Check sheet for the drawn part. Datum: minimum x, y, z corner. Units: mm. Coordinates: 2 decimals unless noted, no trailing zeros. Write each loop counter-clockwise with the first axis right and the second up, starting at its lowest first coordinate (ties: lowest second). Pieces come first, ordered by that corner, then holes. Notation, with made-up numbers: M 27.5,17 L 61.5,17 A19 cw 61.5,54 Z; hole C 84,51 d7. An arc over 180 degrees is marked long. Answer in a Markdown table with one row per item.
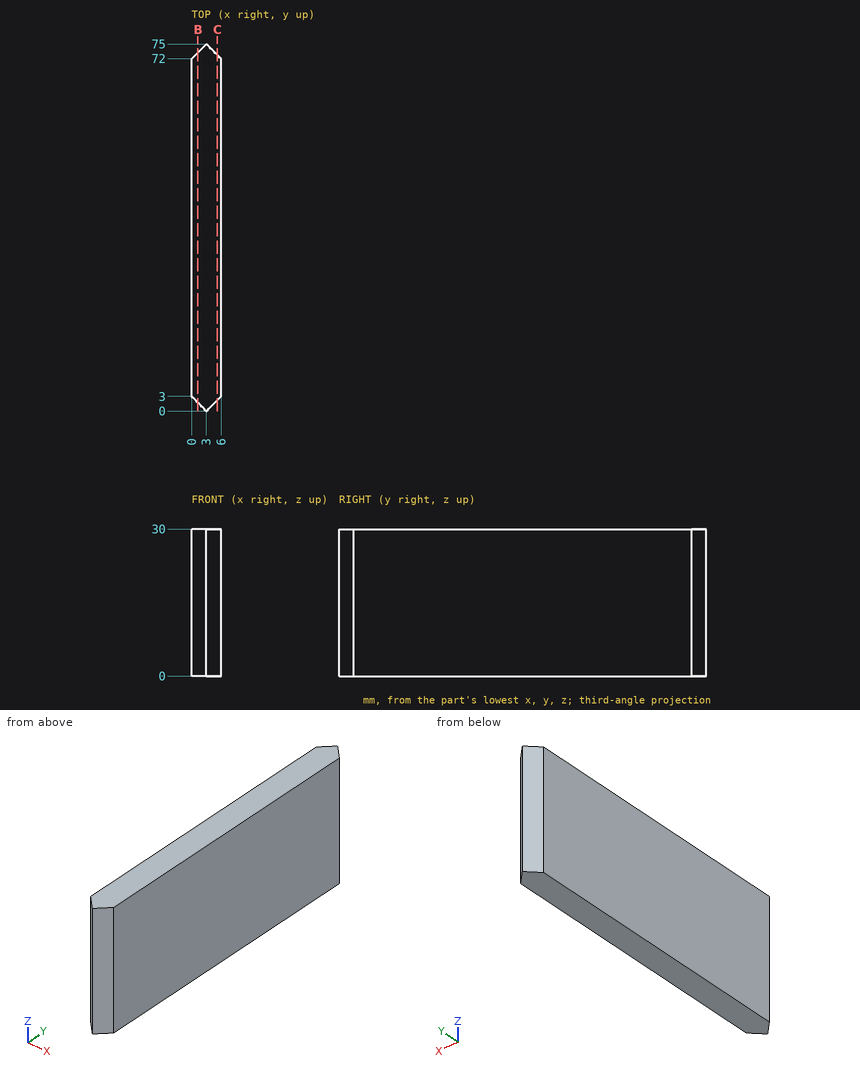
1) Sectioned sample at B-B (x = 1.25). Record the cut outline in (y, z).
Response values:
| item | result |
|---|---|
| outline | M 1.75,0 L 73.25,0 L 73.25,30 L 1.75,30 Z |
2) Depth check by flat-ended pin: pin 1 (3 mm diameter, centred on x = 3.5, z = 7.5, fed in from -Y). Enter the tip coordinate at first touch or a pass-through.
Response values:
| item | result |
|---|---|
| pin 1 | stops at y = 0 |
3) Sectioned sample at C-C (x = 5.25). Record the cut outline in (y, z), then the cut area to 4 significant figures.
Response values:
| item | result |
|---|---|
| outline | M 2.25,0 L 72.75,0 L 72.75,30 L 2.25,30 Z |
| area | 2,115 mm² |
4) Thickness scan on L1, parallel to Y at x = 1, z = 19; L2, parallel to Y at x = 2, z = 22. Record the ranges inside material, lowest first. Write a range as [from, to].
Response values:
| item | result |
|---|---|
| L1 | y = [2, 73] |
| L2 | y = [1, 74] |
